Input: dimensioned drawing with shaded views. Units: mm. Origin: part minimum x, y, z. A direction names the side the tool comes from. Give positions to 0.01 mm unless a question says otherwise; leave off trailing zeros. Loops run counter-clockwise (first coordinate to the right, second up) from the corner with the lowest first, then second, coordinate; pieces in that order, holes last. Notation, with made-up numbers: (26, -16) -> (31, -16) arc R8 ccw to (31, -4) -> close; hole circle Ø5 at (82, -31.5). An arc over 180 degrees is marked (long way). Answer in a Markdown table with one row per item. Add a question column.
1) First-contact query: P1, Ø8, axis at x = 2.5, z = 51, coming from the -Y side; P2, Ø4, axis at x = 10.5, z = 18, coming from the -Y side; P3, Ø1, axis at x = 13, z = 72, coming from the -Y side; P4, Ø2.5, axis at x = 8.5, y = 8.5, coming from the -Z side. Flat tips, straight axial feed; report the tip coordinate or a pass-through.
2) Access query for the marked faces 1 and 2. Directions: +Z, -Z, +X, -X, +Y, -Y. A direction counts if a zero-diameter tool reaches every point of the face in a straight line with its end or side. Return the directions, or none.
3) Section query A-A (y = 8.5). Return the cut outline in (x, z).
4) Section query C-C (z = 48). Return the cut outline in (x, y), plus the area to 3 significant figures.
5) Section query D-D (x = 1.75). Return the cut outline in (y, z), plus the area to 3 significant figures.
6) Line query: line 1 (Y direction, x = 8.5, z = 27); line 2 (Z direction, x = 3, y = 7.5); line 3 (Z direction, x = 4.75, y = 10.75). Output: solid intervals per line, ascending. Write a range as from..to.
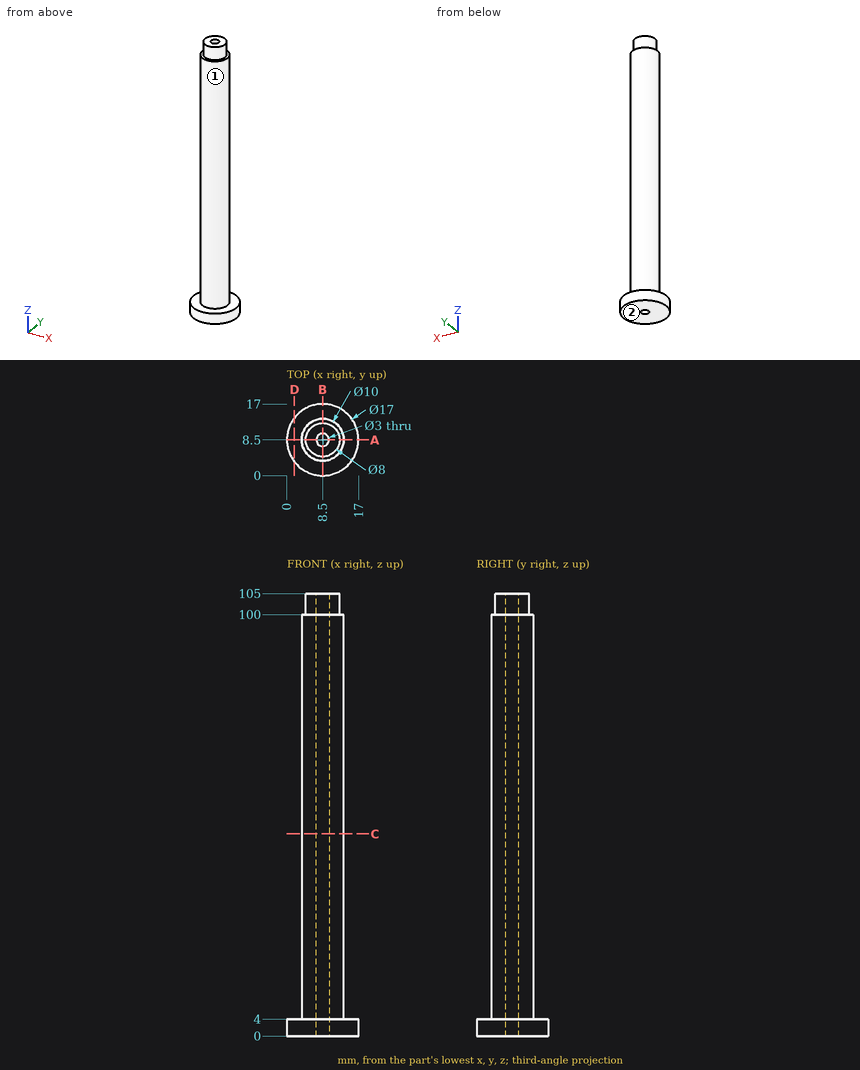
Evaluation:
| question | item | result |
|---|---|---|
| 1 | P1 | y = 3.92 |
| 1 | P2 | y = 3.5 |
| 1 | P3 | y = 5.5 |
| 1 | P4 | through |
| 2 | face 1 | +Z |
| 2 | face 2 | -Z, +X, -X, +Y, -Y |
| 3 | outline | (0, 0) -> (7, 0) -> (7, 105) -> (4.5, 105) -> (4.5, 100) -> (3.5, 100) -> (3.5, 4) -> (0, 4) -> close; (10, 0) -> (17, 0) -> (17, 4) -> (13.5, 4) -> (13.5, 100) -> (12.5, 100) -> (12.5, 105) -> (10, 105) -> close |
| 4 | outline | circle Ø10 at (8.5, 8.5); hole circle Ø3 at (8.5, 8.5) |
| 4 | area | 71.5 mm² |
| 5 | outline | (3.33, 0) -> (13.67, 0) -> (13.67, 4) -> (3.33, 4) -> close |
| 5 | area | 41.3 mm² |
| 6 | line 1 | 3.5..7, 10..13.5 |
| 6 | line 2 | 0..4 |
| 6 | line 3 | 0..100 |
